Source: CAD feature listing. Evaluate the final solid. Frame: model axes, mm. A direction names the side the tool comes from. Round coordinates to 2 decimals unless told otherwise and drop trailing zeros. Write each loop counter-clockwise with the first axis right and the second up, starting at its lowest first coordinate (ties: lowest second). Pieces come first, ordered by that corner, then holes.
Autodesk Inventor part; units mm, degrees
ref_plane "YZ Plane" through (0, 0, 0) normal (1, 0, 0) x (0, 1, 0)
ref_plane "XZ Plane" through (0, 0, 0) normal (0, 1, 0) x (-1, 0, 0)
ref_plane "XY Plane" through (0, 0, 0) normal (0, 0, 1) x (1, 0, 0)
sketch "Unit" plane through (0, 0, 0) normal (0, 0, 1) x (1, 0, 0)
  line L0 (17.4453, 22.2497) -> (21.7153, 22.2497)
  line L1 (21.7153, 22.2497) -> (21.7153, 23.2497)
  line L2 (21.7153, 23.2497) -> (23.4453, 23.2497)
  line L3 (21.7153, 23.2497) -> (21.7153, 24.9797) construction
  line L4 (23.4453, 23.2497) -> (23.4453, 22.6997)
  line L5 (23.4453, 22.6997) -> (25.4453, 22.6997)
  line L6 (25.4453, 22.6997) -> (25.4453, 23.2497)
  line L7 (25.4453, 23.2497) -> (27.1753, 23.2497)
  line L8 (27.1753, 23.2497) -> (27.1753, 22.2497)
  line L9 (27.1753, 22.2497) -> (31.4453, 22.2497)
  line L10 (26.3953, 20.7497) -> (22.4953, 20.7497) construction
  line L11 (22.4953, 20.7497) -> (22.4953, 18.7497) construction
  line L12 (22.4953, 18.7497) -> (26.3953, 18.7497) construction
  line L13 (26.3953, 18.7497) -> (26.3953, 20.7497) construction
  line L14 (26.3953, 20.7497) -> (22.4953, 18.7497) construction
  line L15 (22.4953, 20.7497) -> (26.3953, 18.7497) construction
  point P0 (20.0288, 26.7181)
  point P1 (24.4453, 19.7497)
  dimension "d17" = 2
  dimension "d31" = 110
  dimension "d32" = 0
  dimension "d33" = 2
  dimension "d34" = 20
  dimension "d35" = 20
  dimension "d36" = 1.5
  dimension "d37" = 20.3526
  dimension "d2" = 1
  dimension "d3" = 1.73
  dimension "d4" = 0.55
  dimension "d5" = 2
  dimension "d6" = 1.73
  dimension "d7" = 1
  dimension "d12" = 3.9
  dimension "d13" = 2
  dimension "d14" = 1.5
  dimension "d40" = 14
  dimension "d102" = 4.27
sketch "Anchor" plane through (0, 0, 0) normal (0, 0, 1) x (1, 0, 0)
  line L0 (2, 0) -> (2, 1.875)
  line L1 (2, 0) -> (3, 0) construction
  line L2 (2.125, 2) -> (4.875, 2)
  line L3 (5, 1.875) -> (5, 0)
  line L4 (5, 2) -> (7, 2) construction
  line L5 (0, 0) -> (2, 0)
  line L6 (5, 0) -> (7, 0)
  arc A0 (2.125, 2) -> (2, 1.875) centre (2.125, 1.875) ccw
  arc A1 (5, 1.875) -> (4.875, 2) centre (4.875, 1.875) ccw
  point P0 (9.1321, -0.6227)
  point P1 (2, 2)
  dimension "d69" = 15
  dimension "d45" = 2
  dimension "d46" = 2
  dimension "d47" = 3
  dimension "d48" = 2
  dimension "d60" = 2
  dimension "d67" = 0.125
sketch "Esquisse2" plane through (0, 0, 0) normal (0, 0, 1) x (1, 0, 0)
  line L0 (-10.7801, -14.9425) -> (-8.7801, -14.9425)
  line L1 (-10.7801, -13.9425) -> (-10.7801, -14.9425)
  line L2 (3.2199, -13.9425) -> (3.2199, -14.9425)
  line L3 (-8.7801, -14.9425) -> (-8.7801, -11.6425)
  line L4 (1.2199, -11.6425) -> (1.2199, -14.9425)
  line L5 (1.2199, -14.9425) -> (3.2199, -14.9425)
  line L6 (-8.7801, -11.6425) -> (1.2199, -11.6425)
  line L7 (-10.7801, -11.9425) -> (-12.6551, -11.9425)
  line L8 (-10.7801, -11.9425) -> (-10.7801, -10.9425) construction
  line L9 (-12.7801, -11.8175) -> (-12.7801, -9.0675)
  line L10 (-12.6551, -8.9425) -> (-10.7801, -8.9425)
  line L11 (-12.7801, -8.9425) -> (-12.7801, -6.9425) construction
  line L12 (-10.7801, -13.9425) -> (-10.7801, -11.9425)
  line L13 (-10.7801, -8.9425) -> (-10.7801, -6.9425)
  arc A0 (-12.7801, -11.8175) -> (-12.6551, -11.9425) centre (-12.6551, -11.8175) ccw
  arc A1 (-12.6551, -8.9425) -> (-12.7801, -9.0675) centre (-12.6551, -9.0675) ccw
  line L14 (3.2199, -8.9425) -> (5.0949, -8.9425)
  line L15 (3.2199, -8.9425) -> (3.2199, -9.9425) construction
  line L16 (5.2199, -9.0675) -> (5.2199, -11.8175)
  line L17 (5.0949, -11.9425) -> (3.2199, -11.9425)
  line L18 (5.2199, -11.9425) -> (5.2199, -13.9425) construction
  line L19 (3.2199, -6.9425) -> (3.2199, -8.9425)
  line L20 (3.2199, -11.9425) -> (3.2199, -13.9425)
  arc A2 (5.2199, -9.0675) -> (5.0949, -8.9425) centre (5.0949, -9.0675) ccw
  arc A3 (5.0949, -11.9425) -> (5.2199, -11.8175) centre (5.0949, -11.8175) ccw
  line L21 (-10.7801, -6.9425) -> (-6.5101, -6.9425)
  line L22 (-6.5101, -6.9425) -> (-6.5101, -5.9425)
  line L23 (-6.5101, -5.9425) -> (-4.7801, -5.9425)
  line L24 (-6.5101, -5.9425) -> (-6.5101, -4.2125) construction
  line L25 (-4.7801, -5.9425) -> (-4.7801, -6.4925)
  line L26 (-4.7801, -6.4925) -> (-2.7801, -6.4925)
  line L27 (-2.7801, -6.4925) -> (-2.7801, -5.9425)
  line L28 (-2.7801, -5.9425) -> (-1.0501, -5.9425)
  line L29 (-1.0501, -5.9425) -> (-1.0501, -6.9425)
  line L30 (-1.0501, -6.9425) -> (3.2199, -6.9425)
  line L31 (-1.8301, -8.4425) -> (-5.7301, -8.4425) construction
  line L32 (-5.7301, -8.4425) -> (-5.7301, -10.4425) construction
  line L33 (-5.7301, -10.4425) -> (-1.8301, -10.4425) construction
  line L34 (-1.8301, -10.4425) -> (-1.8301, -8.4425) construction
  line L35 (-1.8301, -8.4425) -> (-5.7301, -10.4425) construction
  line L36 (-5.7301, -8.4425) -> (-1.8301, -10.4425) construction
  point P0 (0, 0)
  point P1 (3.2199, -6.9425)
  point P2 (-10.7801, -6.9425)
  point P3 (-10.7803, -12.8535)
  point P4 (3.2197, -12.8535)
  dimension "d101" = 14
  dimension "d97" = 4.7
  dimension "d98" = 8
  dimension "d99" = 2
  dimension "d100" = 10
extrude "Extrusion1" add sketch "Esquisse2" along normal blind 2
equation "\"d35\" = d34"
equation "\"d6\" = d3"
equation "\"d7\" = d2"
equation "\"d13\" = sheet_thickness"
equation "\"d48\" = sheet_thickness"
equation "\"d99\" = safe_distance"
equation "\"d71\" = sheet_thickness"
properties part number "extra_switch_support" material "Acier inoxydable"
1) Contact query for flat-ended pins moving along their axis: P1, Ø0.8, axis at y = -6.5, z = 1, coming from the -X side; P2, Ø0.5, axis at y = -6, z = 1, coming from the +X side; P3, Ø1, axis at y = -13, z = 0.5, coming from the -X side. Output: stop coordinate, or through.
Taken from the geometry:
P1: stops at x = -6.51
P2: stops at x = -1.05
P3: stops at x = -10.78
2) Material intervals for line 1 (X direction, y = -12, z = 1.4); line 2 (X direction, y = -11.75, z = 0.6); line 3 (Y direction, x = -3.75, z = 1.8), sorted ascending.
Taken from the geometry:
line 1: x = -10.78 to -8.78, 1.22 to 3.22
line 2: x = -12.78 to -8.78, 1.22 to 5.22
line 3: y = -11.64 to -6.49
3) Reachability of faces 1 (the face through (-4, -6.492, 1)), 2 (the face through (-8.78, -13, 1)), 3 (the face through (4, -8.942, 1)) from +Z, -Z, +X, -X, +Y, -Y: full face, straight path, thin tool, end or side. Return the list, or none.
Taken from the geometry:
face 1: +Z, -Z, +Y
face 2: +Z, -Z, -Y
face 3: +Z, -Z, +X, +Y
4) Section query A-A on y = -13.5. Return the cut outline in (x, z).
Taken from the geometry:
outline: (-10.78, 0) - (-8.78, 0) - (-8.78, 2) - (-10.78, 2) - close; (1.22, 0) - (3.22, 0) - (3.22, 2) - (1.22, 2) - close
5) Section query C-C on x = -6.25. Return the cut outline in (y, z), then the cut area to 3 significant figures.
Taken from the geometry:
outline: (-11.64, 0) - (-5.94, 0) - (-5.94, 2) - (-11.64, 2) - close
area: 11.4 mm2
6) Section query D-D on y = -8.5. Return the cut outline in (x, z).
Taken from the geometry:
outline: (-10.78, 0) - (3.22, 0) - (3.22, 2) - (-10.78, 2) - close
